Work out the finished part from the listing and answer in its coordinate system (mm). A direction names the side the tool comes from. Round coordinates to 2 decimals unless told otherwise and drop trailing zeros. Loops run counter-clockwise (first coordinate to the right, second up) from the corner with the lowest first, then second, coordinate; pieces in that order, holes last. Notation, with made-up numbers: (30.5, 51) - (56.5, 51) arc R27 cw to (56.5, 68) - close; hole circle Ø1 at (-25, 80.5). An arc over 180 degrees is marked (long way). Answer as CSV lines item,"result". Start each with the question number.
```python
from build123d import *

# Parameters (mm, degrees)
F0_W     = 195.4201161861
F0_H     = 105.9125140309
F1_DEPTH = 8.636
F2_W     = 185.3469088674
F2_H     = 95.2637046576
F3_DEPTH = 1.016
F4_R     = 3.556
F5_DEPTH = 1.016


# Not quite as in the source:
# - a feature names something its author has since deleted; it is built from what else it names


with BuildPart() as f1:
    # F0 (on Front) → F1 (new body)
    with BuildSketch(Plane.XZ):
        with Locations((2.4463534355, -2.8780587018)):
            Rectangle(F0_W, F0_H)
    extrude(amount=F1_DEPTH)

    # F2 (on face) → F3 (join)
    with BuildSketch(Plane.XZ.offset(8.636)):
        with Locations((2.4463497102, -2.4463459849)):
            Rectangle(F2_W, F2_H)
    extrude(amount=F3_DEPTH)

    # F4 (on face) → F5 (join)
    with BuildSketch(Plane(origin=(0, 0, 0), x_dir=(-1, 0, 0), z_dir=(0, 1, 0))):
        with Locations((-74.3977949023, 43.7464751303)):
            Circle(F4_R)
        with Locations((-74.6855959296, -52.2783157172)):
            Circle(F4_R)
        with Locations((74.3977874517, -52.2783157172)):
            Circle(F4_R)
        with Locations((74.9733969569, 43.7464751303)):
            Circle(F4_R)
    extrude(amount=F5_DEPTH)


solid = f1.part
```
Item 1: Find the intervals of material crossed by L1, parallel to Z at x = 53.5, y = -8.75; L2, parallel to Y at x = -37, z = 13, in increasing order.
Item 2: Section A-A, the plane z = 4.5 is taken. Give the vertices of the cut face in (x, y).
Item 3: Which of the six approach directions +Z, -Z, +X, -X, +Y, -Y give full straight-line access (tool end or side, diameter ignored) to faces 1 (the face through (71.113, 0.501, 42.385)), 2 (the face through (1, -4, -55.834))?
Item 4: A flat-ended cylindrical pin translates along its axis: pin 1 Ø8 at (x, z) = (-66.5, -4.5) entering from +Y. Find the tip coordinate at first contact, or state that the pin passes through.
Item 5: Determine the mould class of faces 3 (the face through (1, -9.652, -2)), 4 (the face through (71.4, 0.5, -53.64)), 5 (the face through (100.156, -4, -4)), 6 (the face through (-95.264, -4, -4)) for opening direction X: pulls with the +X half, pulls with the -X half, needs draft (parallel to the pull), parting line crosses it, or undercut.
Item 6: Section B-B, the plane x = 36.5 is taken. Give the vertices of the cut face in (y, z).
Answer:
1,L1,"z = -50.08 to 45.19"
1,L2,"y = -9.65 to 0"
2,outline,"(-95.26, -8.64) - (-90.23, -8.64) - (-90.23, -9.65) - (95.12, -9.65) - (95.12, -8.64) - (100.16, -8.64) - (100.16, 0) - (-95.26, 0) - close"
3,face 1,"+Y"
3,face 2,"-Z, +X, -X, +Y, -Y"
4,pin 1,"stops at y = 0"
5,face 3,"needs draft"
5,face 4,"undercut"
5,face 5,"pulls with the +X half"
5,face 6,"pulls with the -X half"
6,outline,"(-9.65, -50.08) - (-8.64, -50.08) - (-8.64, -55.83) - (0, -55.83) - (0, 50.08) - (-8.64, 50.08) - (-8.64, 45.19) - (-9.65, 45.19) - close"
